For this review, use the dimensioned drawing (mm, ordinates from the lowest corner) and the shaded views. Coordinates: 2 decimals unless noted, no trailing zeros. Loops run counter-clockwise (first coordinate to the right, second up) from the corner with the lowest first, then second, coordinate; pieces in that order, holes last. Notation, with made-up numbers: M -36.75,-4.5 L -5.75,-4.5 A13 cw -5.75,5.5 Z; hole C -8.75,87 d3. An arc over 180 degrees is marked long. One line per item, written item: value.
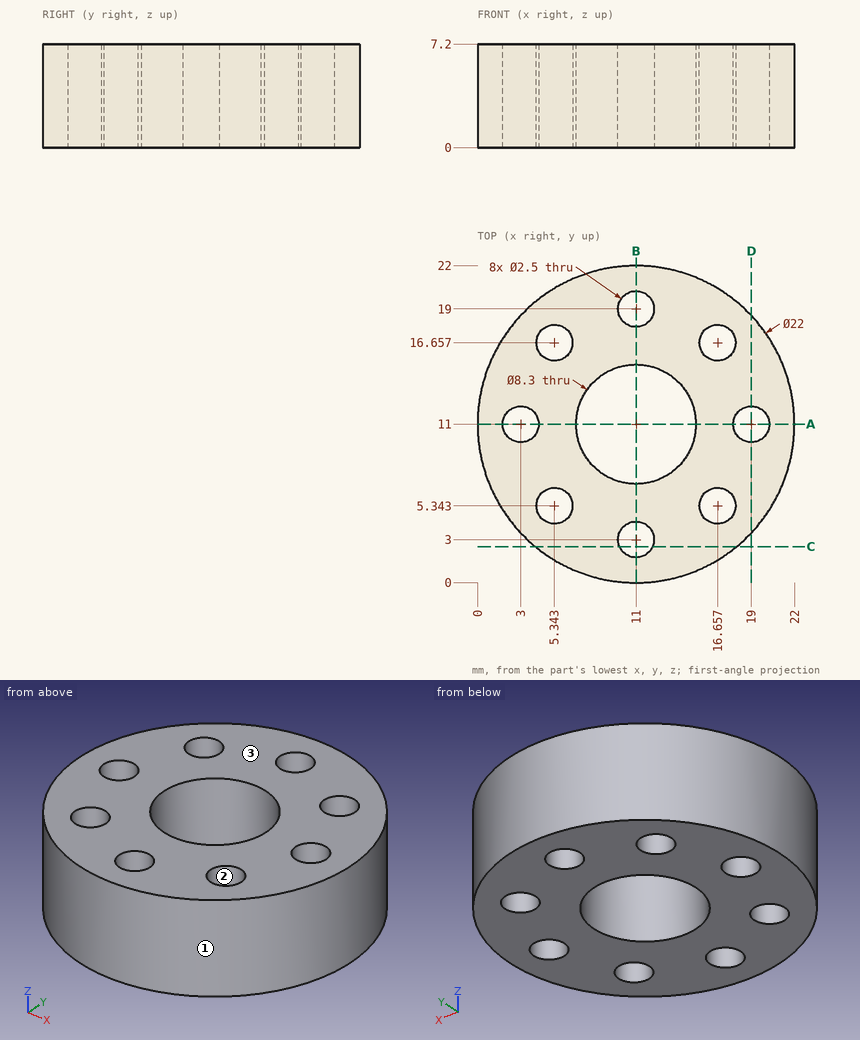
(1) We need section D-D on x = 19. State the section outline as (y, z) points, then the cut area to 3 significant figures.
Reply:
outline: M 3.45,0 L 9.75,0 L 9.75,7.2 L 3.45,7.2 Z; M 12.25,0 L 18.55,0 L 18.55,7.2 L 12.25,7.2 Z
area: 90.7 mm2
(2) We need section C-C on y = 2.5. State the section outline as (x, z) points.
Reply:
outline: M 4.02,0 L 9.85,0 L 9.85,7.2 L 4.02,7.2 Z; M 12.15,0 L 17.98,0 L 17.98,7.2 L 12.15,7.2 Z
(3) We need section A-A on y = 11. State the section outline as (x, z) points.
Reply:
outline: M 0,0 L 1.75,0 L 1.75,7.2 L 0,7.2 Z; M 4.25,0 L 6.85,0 L 6.85,7.2 L 4.25,7.2 Z; M 15.15,0 L 17.75,0 L 17.75,7.2 L 15.15,7.2 Z; M 20.25,0 L 22,0 L 22,7.2 L 20.25,7.2 Z
(4) To check wall thickness, follow line 1 along Y through (x, z) = (11, 4.75); line 2 along Y through (x, z) = (5, 0.75) (1 decimal). State the ranges of each line that lie inside material, in increasing order. Write a range as [from, to].
Reply:
line 1: y = [0, 1.75], [4.25, 6.85], [15.15, 17.75], [20.25, 22]
line 2: y = [1.8, 4.1], [6.5, 15.5], [17.9, 20.2]
(5) Insertion check: pin 1 (1 mm diameter, centred on x = 9, z = 4, fed in from -Y); pin 2 (3 mm diameter, centred on x = 16, z = 2.5, fed in from +Y). Each pin has a flat end and moves straight along its axis. Give the tip position at first contact, or say it passes through.
Reply:
pin 1: stops at y = 0.1
pin 2: stops at y = 21.43
(6) Mouldability with a two-part tool opening along X and no side actions: class the marked faces 1, 2 and 3 as released by +X, released by -X, zero draft, split by the parting line, or undercut.
Reply:
face 1: split by the parting line
face 2: undercut
face 3: zero draft
